```python
from build123d import *

# Parameters (mm, degrees)
ESBO_O1_W                          = 90
ESBO_O1_H                          = 93
RESSALTO_EXTRUS_O1_DEPTH           = 12.7
ESBO_O3_R                          = 32.51
CORTE_EXTRUS_O2_DEPTH              = 66.943460631
CORTE_EXTRUS_O4_REACH              = 67.943
ESBO_O5_W                          = 27.5
ESBO_O5_H                          = 13
CORTE_EXTRUS_O5_REACH              = 67.943
ESBO_O6_W                          = 7
ESBO_O6_H                          = 26.329700269
CORTE_EXTRUS_O6_REACH              = 80.929
ESBO_O7_R                          = 2.5
TALADRO_DE_MARGEN_PARA_00001_D     = 5
TALADRO_DE_MARGEN_PARA_00001_DEPTH = 20
TALADRO_DE_MARGEN_PARA_00001_TIP   = 1.502151548


with BuildPart() as part:
    # Esboço1 → Ressalto-extrusão1 (new body)
    with BuildSketch(Plane(origin=(0, 0, 0), x_dir=(1, 0, 0), z_dir=(0, 1, 0))):
        Rectangle(ESBO_O1_W, ESBO_O1_H)
    extrude(amount=RESSALTO_EXTRUS_O1_DEPTH)

    # Esboço3 → Corte-extrusão2 (cut, through all)
    with BuildSketch(Plane(origin=(0, 12.7, 0), x_dir=(1, 0, 0), z_dir=(0, 1, 0))):
        with Locations(Location((0, 3.5, 0), (0, 0, 270))):
            Circle(ESBO_O3_R)
    extrude(amount=-CORTE_EXTRUS_O2_DEPTH, mode=Mode.SUBTRACT)

    # Esboço5 → Corte-extrusão4 (cut, up to next)
    with BuildSketch(Plane(origin=(0, 12.7, 0), x_dir=(1, 0, 0), z_dir=(0, 1, 0)), mode=Mode.PRIVATE) as corte_extrus_o4_sk1:
        with Locations((31.25, -40)):
            Rectangle(ESBO_O5_W, ESBO_O5_H)
    corte_extrus_o4_tool1 = extrude(corte_extrus_o4_sk1.sketch, amount=-CORTE_EXTRUS_O4_REACH, mode=Mode.PRIVATE) & part.part
    # Esboço5 → Corte-extrusão4 (cut, up to next)
    with BuildSketch(Plane(origin=(0, 12.7, 0), x_dir=(1, 0, 0), z_dir=(0, 1, 0)), mode=Mode.PRIVATE) as corte_extrus_o4_sk2:
        with Locations((-31.25, -40)):
            Rectangle(ESBO_O5_W, ESBO_O5_H)
    corte_extrus_o4_tool2 = extrude(corte_extrus_o4_sk2.sketch, amount=-CORTE_EXTRUS_O4_REACH, mode=Mode.PRIVATE) & part.part
    add(corte_extrus_o4_tool1.solids().sort_by_distance((31.25, 12.7, 40))[0], mode=Mode.SUBTRACT)
    add(corte_extrus_o4_tool2.solids().sort_by_distance((-31.25, 12.7, 40))[0], mode=Mode.SUBTRACT)

    # Esboço6 → Corte-extrusão5 (cut, up to next)
    with BuildSketch(Plane(origin=(0, 12.7, 0), x_dir=(1, 0, 0), z_dir=(0, 1, 0)), mode=Mode.PRIVATE) as corte_extrus_o5_sk1:
        with Locations((0, -33.335149866)):
            Rectangle(ESBO_O6_W, ESBO_O6_H)
    corte_extrus_o5_tool1 = extrude(corte_extrus_o5_sk1.sketch, amount=-CORTE_EXTRUS_O5_REACH, mode=Mode.PRIVATE) & part.part
    add(corte_extrus_o5_tool1.solids().sort_by_distance((0, 12.7, 33.33515))[0], mode=Mode.SUBTRACT)

    # Corte-extrusão6: up to this face of the body (flat: up to its plane)
    corte_extrus_o6_end = Plane(part.part.faces().sort_by_distance((17.5, 6.35, 40))[0])
    # Esboço7 → Corte-extrusão6 (cut, up to the picked face)
    with BuildSketch(Plane.ZY.offset(17.5), mode=Mode.PRIVATE) as corte_extrus_o6_sk1:
        with Locations((41.5, 6.35)):
            Circle(ESBO_O7_R)
    corte_extrus_o6_tool1 = split(extrude(corte_extrus_o6_sk1.sketch, amount=-CORTE_EXTRUS_O6_REACH, mode=Mode.PRIVATE), bisect_by=corte_extrus_o6_end, keep=Keep.BOTH, mode=Mode.PRIVATE)
    add(corte_extrus_o6_tool1.solids().sort_by(Axis((-17.5, 6.35, 41.5), (1, 0, 0)))[0], mode=Mode.SUBTRACT)

    # Taladro de margen para #00001
    with Locations(Plane(origin=(0, 0, -46.5), x_dir=(-1, 0, 0), z_dir=(0, 0, -1))):
        with Locations((-40, 6.35), (-25, 6.35), (40, 6.35), (25, 6.35)):
            Hole(TALADRO_DE_MARGEN_PARA_00001_D / 2, depth=TALADRO_DE_MARGEN_PARA_00001_DEPTH)
            with Locations((0, 0, -(TALADRO_DE_MARGEN_PARA_00001_DEPTH + TALADRO_DE_MARGEN_PARA_00001_TIP / 2))):  # 118° drill point
                Cone(0, TALADRO_DE_MARGEN_PARA_00001_D / 2, TALADRO_DE_MARGEN_PARA_00001_TIP, mode=Mode.SUBTRACT)


solid = part.part
```
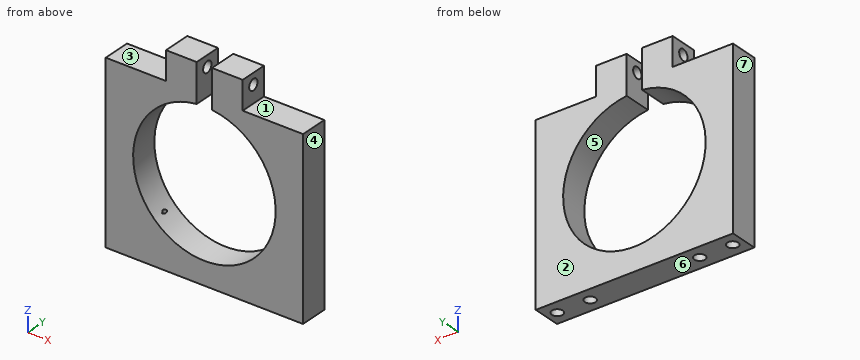
Part model, mm, in its own coordinate system. Face numbers are marked on the shaded views. A direction names the side the tool comes from. Coordinates: 2 decimals unless noted, no trailing zeros. Order: outer loops, then holes, each group sorted by start corner. A loop starts at its lowest first (then second) coordinate and runs counter-clockwise, first axis right, second up. Notation, with made-up numbers: (31.25, -18) - (87.25, -18) arc R18 ccw to (87.25, -10) - close; hole circle Ø10 at (-22.75, 4). An arc over 180 degrees is marked (long way). Return JSON: item names as keys, results as strings. Group by question number.
Item 1: Which spindle directions (+Z, -Z, +X, -X, +Y, -Y) get a long thin tool onto all of the face, cutting with end or side? Do the marked faces 1, 2 and 3. Say none if no direction does.
Item 2: Drill centre lines: probe 1 along X at (y, z) = (6.25, -37); probe 2 along X at (y, z) = (6.35, -32); probe 3 along X at (y, z) = (8.5, -38). Where is each one in solid material? Low to high. Write a range as from..to.
Item 3: Cut at A-A (x = 16). List the corners of the cut face in (y, z).
Item 4: Pull direction X, two halves, no side cores. Call the marked faces 4, 5, 6 and 7: pulls with the +X half, pulls with the -X half, needs draft (parallel to the pull), parting line crosses it, or undercut.
Item 5: Pin check, flat tips, straight feed: pin 1 (6 mm diameter, centred on x = 30, z = 5.5, fed in from +Y); pin 2 (6 mm diameter, centred on x = 31.5, y = 5, fed in from +Z); pin 3 (3 mm diameter, centred on x = 25, y = 6.35, fed in from -Z). Stop position of each tip, or through.
Item 6: Cut at C-C (y = 10.5). List the corners of the cut face in (x, z), plus the area to 3 significant figures.
Item 7: Cut at D-D (x = 0). List the corners of the cut face in (y, z), plus the area to 3 significant figures.
Item 8: Cut at B-B (z = -15). List the corners of the cut face in (x, y).
Check values:
{
 "1": {"face 1": "+Z, +X, +Y, -Y", "face 2": "+Z, -Z, +X, -X, +Y", "face 3": "+Z, -X, +Y, -Y"},
 "2": {"probe 1": "x = -45..-42.5, -37.5..-27.5, -22.5..22.5, 27.5..37.5, 42.5..45", "probe 2": "x = -45..-42.5, -37.5..-27.5, -22.5..-15.64, 15.64..22.5, 27.5..37.5, 42.5..45", "probe 3": "x = -45..-41.28, -38.72..-26.28, -23.72..23.72, 26.28..38.72, 41.28..45"},
 "3": {"outline": "(0, -46.5) - (12.7, -46.5) - (12.7, -31.8) - (0, -31.8) - close; (0, 24.8) - (12.7, 24.8) - (12.7, 46.5) - (0, 46.5) - close; hole circle Ø5 at (6.35, 41.5)"},
 "4": {"face 4": "pulls with the +X half", "face 5": "undercut", "face 6": "needs draft", "face 7": "pulls with the -X half"},
 "5": {"pin 1": "stops at y = 12.7", "pin 2": "stops at z = 33.5", "pin 3": "stops at z = -25.9"},
 "6": {"outline": "(-45, -46.5) - (45, -46.5) - (45, 33.5) - (17.5, 33.5) - (17.5, 46.5) - (3.5, 46.5) - (3.5, 28.82) arc R32.51 cw (long way) to (-3.5, 28.82) - (-3.5, 46.5) - (-17.5, 46.5) - (-17.5, 33.5) - (-45, 33.5) - close", "area": "4,210 mm2"},
 "7": {"outline": "(0, -46.5) - (12.7, -46.5) - (12.7, -36.01) - (0, -36.01) - close", "area": "133 mm2"},
 "8": {"outline": "(-45, 0) - (-30.41, 0) - (-30.41, 12.7) - (-45, 12.7) - close; (30.41, 0) - (45, 0) - (45, 12.7) - (30.41, 12.7) - close"}
}
